Geometry: final body of the model. Coordinates: model frame, mm. Face numbers are marked on the shaded views. A direction names the side the tool comes from. Round coordinates to 2 decimals unless told otherwise and drop trailing zeros. Order: outer loops, then holes, each group sorted by start corner. A loop starts at its lowest first (then second) coordinate and runs counter-clockwise, first axis right, second up. Notation, with made-up numbers: (-26.75, 78.5) -> (15.25, 78.5) arc R23 ccw to (15.25, 96.5) -> close; hole circle Ø6 at (-33, 78.25). An arc over 180 degrees is marked (long way). Put each result on its own line as item: value.
```python
from build123d import *

# Parameters (mm, degrees)
BOSS_EXTRUDE1_DEPTH = 27.94
BOSS_EXTRUDE3_DEPTH = 25.4
SKETCH5_R           = 19.06504515
BOSS_EXTRUDE4_DEPTH = 10.16
SKETCH6_R           = 7
BOSS_EXTRUDE5_DEPTH = 76.2


with BuildPart() as part:
    # Sketch1 → Boss-Extrude1 (new body)
    with BuildSketch(Plane(origin=(0, 0, 0), x_dir=(1, 0, 0), z_dir=(0, 1, 0))):
        with BuildLine():
            Line((-5.3, -3.217204022), (5.3, -3.217204022))
            ThreePointArc((5.3, -3.217204022), (0, 3.217204022), (-5.3, -3.217204022))
        make_face()
    extrude(amount=BOSS_EXTRUDE1_DEPTH)

    # Sketch4 → Boss-Extrude3 (add)
    with BuildSketch(Plane(origin=(0, 27.94, 0), x_dir=(1, 0, 0), z_dir=(0, 1, 0))):
        with BuildLine():
            Line((5.3, -3.217204022), (-5.3, -3.217204022))
            ThreePointArc((-5.3, -3.217204022), (0, -7.582795978), (5.3, -3.217204022))
        make_face()
        with BuildLine():
            Line((-5.3, -3.217204022), (5.3, -3.217204022))
            ThreePointArc((5.3, -3.217204022), (0, 3.217204022), (-5.3, -3.217204022))
        make_face()
    extrude(amount=BOSS_EXTRUDE3_DEPTH)

    # Sketch5 → Boss-Extrude4 (add)
    with BuildSketch(Plane(origin=(0, 53.34, 0), x_dir=(1, 0, 0), z_dir=(0, 1, 0))):
        with Locations((0, -2.182795978)):
            Circle(SKETCH5_R)
    extrude(amount=BOSS_EXTRUDE4_DEPTH)

    # Sketch6 → Boss-Extrude5 (add)
    with BuildSketch(Plane(origin=(0, 63.5, 0), x_dir=(1, 0, 0), z_dir=(0, 1, 0))):
        with Locations((0, -2.182795978)):
            Circle(SKETCH6_R)
    extrude(amount=BOSS_EXTRUDE5_DEPTH)


solid = part.part
```
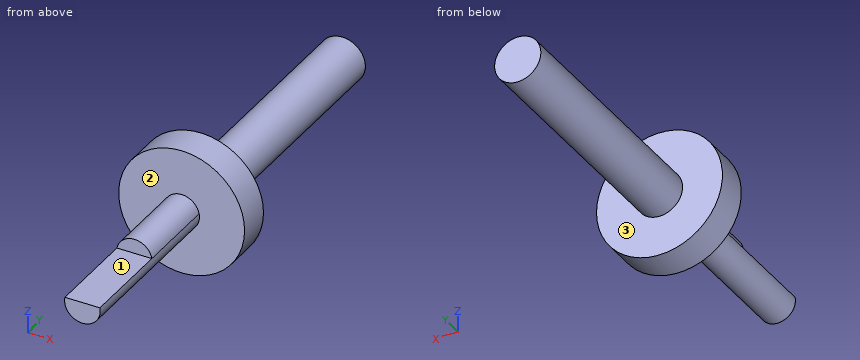
1. Cut plane D-D on y = 111. Return loops of the section in (x, z), and give its area (3 significant figures).
Ans:
outline: circle Ø14 at (0, 2.18)
area: 154 mm²
2. Cut plane A-A on x = 0. Return loops of the section in (y, z).
Ans:
outline: (0, -3.22) -> (53.34, -3.22) -> (53.34, -16.88) -> (63.5, -16.88) -> (63.5, -4.82) -> (139.7, -4.82) -> (139.7, 9.18) -> (63.5, 9.18) -> (63.5, 21.25) -> (53.34, 21.25) -> (53.34, 7.58) -> (27.94, 7.58) -> (27.94, 3.22) -> (0, 3.22) -> close
3. Contact query for flat-ended pins moving along their axis: P1, Ø5, axis at x = 6, y = 75.5, coming from the +Z side (3 decimals); P2, Ø8.5, axis at x = 1, y = 17, coming from the +Z side; P3, Ø5, axis at x = 6.5, z = 10.5, coming from the -Y side. Output: stop coordinate, or through.
Ans:
P1: z = 8.245
P2: z = 3.22
P3: y = 53.34
4. Cut plane B-B on y = 11. Return loops of the section in (x, z), and give its area (3 significant figures).
Ans:
outline: (-5.3, 3.22) arc R5.4 ccw (long way) to (5.3, 3.22) -> close
area: 56.9 mm²
5. Set-up query: the marked faces 1, 2 and 3. Return all of +Z, -Z, +X, -X, +Y, -Y with unobstructed straight access to the full face (end or side cutting, diameter ignored); none if empty.
Ans:
face 1: +Z, +X, -X, -Y
face 2: -Y
face 3: +Y
6. Material intervals for probe 1 along Y at (x, z) = (14, 7.5); probe 2 along Z at (x, y) = (0, 102); probe 3 along X at (y, z) = (57.5, -4), sorted ascending.
Ans:
probe 1: 53.34 to 63.5
probe 2: -4.82 to 9.18
probe 3: -18.03 to 18.03
7. Cut plane C-C on x = 11.5. Return loops of the section in (y, z).
Ans:
outline: (53.34, -13.02) -> (63.5, -13.02) -> (63.5, 17.39) -> (53.34, 17.39) -> close
